Read the model definition and answer for the solid it produces. Units are mm, in the model's axes. Face numbers are marked on the shaded views. Coordinates: 2 decimals unless noted, no trailing zeros. Write each loop counter-clockwise with the first axis right and the second up, starting at its lowest first coordinate (ties: lowest second). Pieces come first, ordered by that corner, then holes.
1) The part is cut by section A-A (y = 5). Determine the outline of the cut face in (x, z), then the cut area to 3 significant figures.
2) This flat-tipped pin is pushed along its axis until it touches: pin 1 Ø4 at (x, y) = (5, 5) entering from +Z. Where does it stop, or does it pass through?
3) The part is cut by section C-C (x = 8.5). Determine the outline of the cut face in (y, z), then the cut area to 3 significant figures.
4) Determine the mould class of the marked faces 1, 2, 3 and 4 for opening direction Y: +Y half, -Y half, draft (parallel to the pull), parting line (faces both ways), or undercut.
5) Find the intervals of material crossed by line 1 (Z direction, x = 8.7, y = 5), in increasing order.
from build123d import *

# Parameters (mm, degrees)
SKETCH_1_W          = 10
SKETCH_1_H          = 10
EXTRUDE_1_DEPTH     = 10
SKETCH_2_R          = 1.5
CUT_EXTRUDE_1_DEPTH = 18.320508076
SKETCH_3_R          = 1.5
CUT_EXTRUDE_2_DEPTH = 18.320508076
SKETCH_4_R          = 1.5
CUT_EXTRUDE_3_DEPTH = 18.320508076


with BuildPart() as part:
    # 草图1 → 凸台-拉伸1 (new body)
    with BuildSketch(Plane.XY):
        with Locations((5, 5)):
            Rectangle(SKETCH_1_W, SKETCH_1_H)
    extrude(amount=EXTRUDE_1_DEPTH)

    # 草图2 → 切除-拉伸1 (cut, through all)
    with BuildSketch(Plane.XY.offset(10)):
        with Locations((5, 5)):
            Circle(SKETCH_2_R)
    extrude(amount=-CUT_EXTRUDE_1_DEPTH, mode=Mode.SUBTRACT)

    # 草图3 → 切除-拉伸2 (cut, through all)
    with BuildSketch(Plane.ZY):
        with Locations((5, 5)):
            Circle(SKETCH_3_R)
    extrude(amount=-CUT_EXTRUDE_2_DEPTH, mode=Mode.SUBTRACT)

    # 草图4 → 切除-拉伸3 (cut, through all)
    with BuildSketch(Plane(origin=(0, 10, 0), x_dir=(1, 0, 0), z_dir=(0, 1, 0))):
        with Locations(Location((5, -5, 0), (0, 0, 270))):
            Circle(SKETCH_4_R)
    extrude(amount=-CUT_EXTRUDE_3_DEPTH, mode=Mode.SUBTRACT)


solid = part.part
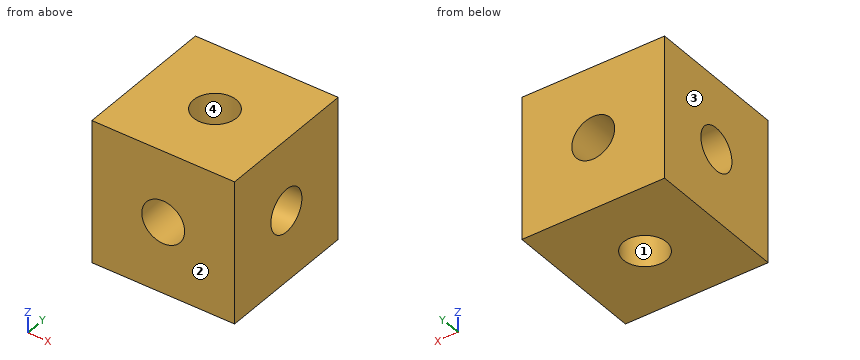
Reported:
1. outline: (0, 0) - (3.5, 0) - (3.5, 3.5) - (0, 3.5) - close; (0, 6.5) - (3.5, 6.5) - (3.5, 10) - (0, 10) - close; (6.5, 0) - (10, 0) - (10, 3.5) - (6.5, 3.5) - close; (6.5, 6.5) - (10, 6.5) - (10, 10) - (6.5, 10) - close
1. area: 49.0 mm2
2. pin 1: stops at z = 10
3. outline: (0, 0) - (10, 0) - (10, 10) - (0, 10) - close; hole circle Ø3 at (5, 5)
3. area: 92.9 mm2
4. face 1: undercut
4. face 2: -Y half
4. face 3: draft
4. face 4: undercut
5. line 1: z = 0 to 3.5, 6.5 to 10
